```python
from build123d import *

# Parameters (mm, degrees)
F1_DEPTH       = 3
F3_DEPTH       = 3
F5_DEPTH       = 3
F6_D           = 4.4
F6_DEPTH       = 80
F6_TIP         = 1.3218933619
F7_D           = 4.4
F7_DEPTH       = 80
F7_TIP         = 1.3218933619
F7_ON_F4_D     = 4.4
F7_ON_F4_DEPTH = 80
F7_ON_F4_TIP   = 1.3218933619
F9_SIZE        = 3
F10_SIZE       = 5


with BuildPart() as f1:
    # F0 (on Front) → F1 (new body)
    with BuildSketch(Plane.XZ):
        Polygon((-83.1050851941, 50), (-103.1050851941, 50), (-103.1050851941, 0), (-53.1050851941, 0), (-53.1050851941, 20), (-83.1050851941, 20), align=None)
    extrude(amount=F1_DEPTH)

    # F2 (on face) → F3 (join)
    with BuildSketch(Plane(origin=(-103.1050851941, 0, 0), x_dir=(0, -1, 0), z_dir=(-1, 0, 0))):
        Polygon((0, 0), (0, 50), (-17, 50), (-17, 20), (-47, 20), (-47, 0), align=None)
    extrude(amount=-F3_DEPTH)

    # F4 (on face) → F5 (join)
    with BuildSketch(Plane(origin=(0, 0, 0), x_dir=(1, 0, 0), z_dir=(0, 0, -1))):
        Polygon((-53.1050851941, -17), (-53.1050851941, 3), (-103.1050851941, 3), (-103.1050851941, -47), (-83.1050851941, -47), (-83.1050851941, -17), align=None)
    extrude(amount=-F5_DEPTH)

    # F6
    with Locations(Plane(origin=(0, 0, 0), x_dir=(1, 0, 0), z_dir=(0, 1, 0))):
        with Locations((-63.1050851941, -12), (-91.1050851941, -40), (-91.1050851941, -12)):
            Hole(F6_D / 2, depth=F6_DEPTH)
            with Locations((0, 0, -(F6_DEPTH + F6_TIP / 2))):  # 118° drill point
                Cone(0, F6_D / 2, F6_TIP, mode=Mode.SUBTRACT)

    # F7
    with Locations(Plane(origin=(-103.1050851941, 0, 0), x_dir=(0, -1, 0), z_dir=(-1, 0, 0))):
        with Locations((-9, 40.2020410289), (-37, 12), (-9, 12)):
            Hole(F7_D / 2, depth=F7_DEPTH)
            with Locations((0, 0, -(F7_DEPTH + F7_TIP / 2))):  # 118° drill point
                Cone(0, F7_D / 2, F7_TIP, mode=Mode.SUBTRACT)

    # F7 on F4
    with Locations(Plane(origin=(0, 0, 0), x_dir=(1, 0, 0), z_dir=(0, 0, -1))):
        with Locations((-91.1050851941, -9), (-91.1050851941, -37), (-63.1050851941, -9)):
            Hole(F7_ON_F4_D / 2, depth=F7_ON_F4_DEPTH)
            with Locations((0, 0, -(F7_ON_F4_DEPTH + F7_ON_F4_TIP / 2))):  # 118° drill point
                Cone(0, F7_ON_F4_D / 2, F7_ON_F4_TIP, mode=Mode.SUBTRACT)

    # F9
    f9_edges = [f1.edges().sort_by_distance(p)[0] for p in [
        (-76.605085, 0, 3),
        (-100.105085, 23.5, 3),
        (-100.105085, 0, 26.5),
    ]]
    chamfer(f9_edges, length=F9_SIZE)

    # F10
    f10_edges = [f1.edges().sort_by_distance(p)[0] for p in [
        (-53.105085, -1.5, 20),
        (-53.105085, 17, 1.5),
        (-83.105085, 47, 1.5),
        (-101.605085, 47, 20),
        (-83.105085, -1.5, 50),
        (-101.605085, 17, 50),
    ]]
    chamfer(f10_edges, length=F10_SIZE)


solid = f1.part
```
Work out the finished part from the listing and answer in its coordinate system (mm). A direction names the side the tool comes from. Give positions to 0.01 mm unless a question says otherwise; leave off trailing zeros. Loops run counter-clockwise (first coordinate to the right, second up) from the corner with the lowest first, then second, coordinate; pieces in that order, holes last. Notation, with made-up numbers: (87.25, -19.5) -> (146.25, -19.5) arc R20 cw to (146.25, -15.5) -> close; hole circle Ø11 at (10.5, 26.5). An arc over 180 degrees is marked (long way). Write item = value, one per line. Start each with the question number.
(1) The mould has two halves that part along Z. Classify faces 4 (the cylindrical face through (-60.907, -1.521, 11.903)), 5 (the flat face through (-55.64, -1.479, 17.535)), 6 (the flat face through (-103.105, 16.8, 19.8)), 7 (the cylindrical face through (-101.584, 8.523, 38.054)): +Z half, -Z half, draft (parallel to the pull), parting line (faces both ways), or undercut.
(2) Find the intervals of material crossed by probe 1 along Z at (x, y) = (-101.95, 37); probe 2 along Y at (x, z) = (-100.5, 33.5); probe 3 along Z at (x, y) = (-75.5, 13), in increasing order. Write a range as from..to.
(3) Which of the six approach directions +Z, -Z, +X, -X, +Y, -Y give full straight-line access (tool end or side, diameter ignored) to faces 1 (the flat face through (-83.105, 30, 1)), 2 (the flat face through (-102, 17, 33)), 3 (the flat face through (-75, 1, 5))?
(4) Find section D-D on y = 23.5. Give the vertices of the cut face in (x, z), and give its area (4 significant figures).
(5) Find section C-C on x = -74.5. Give the vertices of the cut face in (y, z), and give its area (4 significant figures).
(6) Find section A-A on z = 12. Give the vertices of the cut face in (x, y).
(7) Find section B-B on y = 37. Give the vertices of the cut face in (x, z), and give its area (3 significant figures).
(8) Given pin 1 Ø13 at (y, z) = (29, 20.5) entering from +X; pin 2 Ø3.5 at (y, z) = (9, 12) entering from +X; pin 3 Ø2.5 at (x, z) = (-72, 1.5) entering from +Y; pin 4 Ø2.5 at (x, y) = (-102, 31) entering from +Z, each flat-ended and moving along its own axis, determine where each tip first touches the part or whether it passes through.
From the geometry:
q1.face_4 = undercut
q1.face_5 = +Z half
q1.face_6 = draft
q1.face_7 = undercut
q2.probe_1 = 0..9.8, 14.2..20
q2.probe_2 = -3..17
q2.probe_3 = 0..3
q3.face_1 = +Z, -Z, +X, +Y
q3.face_2 = +Z, +X, -X, +Y
q3.face_3 = +Z, +X, +Y
q4.outline = (-103.11, 0) -> (-83.11, 0) -> (-83.11, 3) -> (-97.11, 3) -> (-100.11, 6) -> (-100.11, 20) -> (-103.11, 20) -> close
q4.area = 115.5 mm^2
q5.outline = (-3, 0) -> (17, 0) -> (17, 3) -> (3, 3) -> (0, 6) -> (0, 20) -> (-3, 20) -> close
q5.area = 115.5 mm^2
q6.outline = (-103.11, -3) -> (-93.31, -3) -> (-93.31, 0) -> (-97.11, 0) -> (-100.11, 3) -> (-100.11, 6.8) -> (-103.11, 6.8) -> close; (-103.11, 11.2) -> (-100.11, 11.2) -> (-100.11, 34.8) -> (-103.11, 34.8) -> close; (-103.11, 39.2) -> (-100.11, 39.2) -> (-100.11, 47) -> (-103.11, 47) -> close; (-88.91, -3) -> (-65.31, -3) -> (-65.31, 0) -> (-88.91, 0) -> close; (-60.91, -3) -> (-53.11, -3) -> (-53.11, 0) -> (-60.91, 0) -> close
q7.outline = (-103.11, 0) -> (-93.31, 0) -> (-93.31, 3) -> (-97.11, 3) -> (-100.11, 6) -> (-100.11, 9.8) -> (-103.11, 9.8) -> close; (-103.11, 14.2) -> (-100.11, 14.2) -> (-100.11, 20) -> (-103.11, 20) -> close; (-88.91, 0) -> (-83.11, 0) -> (-83.11, 3) -> (-88.91, 3) -> close
q7.area = 89.1 mm^2
q8.pin_1 = -100.11
q8.pin_2 = through
q8.pin_3 = 17
q8.pin_4 = 20
